from build123d import *

# Parameters (mm, degrees)
F0_W      = 72
F0_H      = 15
F1_DEPTH  = 3.8
F3_DEPTH  = 72
F4_R      = 5
F5_W      = 36
F5_H      = 2
F6_DEPTH  = 1
F7_R      = 0.99999
F10_DEPTH = 4
F11_R     = 2
F12_R     = 1


# Not quite as in the source:
# - a fillet or chamfer is up to 0.001 mm smaller than in the source, because OpenCascade refuses the exact size
# - a pattern or mirror of a feature is missing from the dataset's text; its kind, count and spacing are read off the source's solid


with BuildPart() as f1:
    # F0 (on Top) → F1 (new body)
    with BuildSketch(Plane.XY):
        Rectangle(F0_W, F0_H)
    extrude(amount=F1_DEPTH)

    # F2 (on face) → F3 (join)
    with BuildSketch(Plane.YZ.offset(36)):
        with BuildLine():
            Line((7.5, 7), (5.4598534779, 7))
            ThreePointArc((5.4598534779, 7), (0, 4.8), (-5.4598534779, 7))
            Line((-5.4598534779, 7), (-7.5, 7))
            Line((-7.5, 7), (-7.5, 3.8))
            Line((-7.5, 3.8), (7.5, 3.8))
            Line((7.5, 3.8), (7.5, 7))
        make_face()
    extrude(amount=-F3_DEPTH)

    # F4
    f4_edges = [f1.edges().sort_by_distance(p)[0] for p in [
        (-36, -7.5, 3.5),
        (36, -7.5, 3.5),
        (36, 7.5, 3.5),
        (-36, 7.5, 3.5),
    ]]
    fillet(f4_edges, radius=F4_R)

    # F5 (on face) → F6 (cut)
    with BuildSketch(Plane(origin=(0, 0, 0), x_dir=(1, 0, 0), z_dir=(0, 0, -1))):
        Rectangle(F5_W, F5_H)
    extrude(amount=-F6_DEPTH, mode=Mode.SUBTRACT)

    # F7 (radius 1 in the source; OpenCascade refuses exactly that, so slightly less here)
    f7_edges = [f1.edges().sort_by_distance(p)[0] for p in [
        (0, -1, 1),
        (0, 1, 1),
    ]]
    fillet(f7_edges, radius=F7_R)

    # F9 (on offset) → F10 (cut)
    with BuildSketch(Plane.YZ.offset(16)):
        Polygon((-3.8, 0), (-1.8, 0), (-1.8, 1.8), (0, 1.8), (1.8, 1.8), (1.8, 0), (3.8, 0), (3.8, 3.8), (0, 3.8), (-3.8, 3.8), align=None)
    f10 = extrude(amount=-F10_DEPTH, mode=Mode.SUBTRACT)

    # F10_copies: F10 across plane
    add(f10.mirror(Plane(origin=(0, 0, 0), x_dir=(0, 0, -1), z_dir=(-1, 0, 0))), mode=Mode.SUBTRACT)

    # F11
    f11_edges = [f1.edges().sort_by_distance(p)[0] for p in [
        (14, -3.8, 3.8),
        (14, 3.8, 3.8),
        (-14, -3.8, 3.8),
        (-14, 3.8, 3.8),
    ]]
    fillet(f11_edges, radius=F11_R)

    # F12
    f12_edges = [f1.edges().sort_by_distance(p)[0] for p in [
        (14, -1.8, 1.8),
        (14, 1.8, 1.8),
        (-14, 1.8, 1.8),
        (-14, -1.8, 1.8),
    ]]
    fillet(f12_edges, radius=F12_R)


solid = f1.part
The model under review builds one solid part; all positions refer to its coordinate system, in mm. A direction names the side the tool comes from. Round coordinates to 2 decimals unless told otherwise and drop trailing zeros. Write each loop counter-clockwise with the first axis right and the second up, starting at its lowest first coordinate (ties: lowest second). Pieces come first, ordered by that corner, then holes. Notation, with made-up numbers: M 38.5,63 L 90.5,63 A23 ccw 90.5,99 Z; hole C -16,29.25 d9. An arc over 180 degrees is marked long. Answer as CSV lines item,"result". Start each with the question number.
Q1. Wall thickness on line 1 along X through (y, z) = (-1.75, 2.25); line 2 along Y through (x, z) = (-18, 6.25); line 3 along Y through (x, z) = (17.5, 5.75): over which ranges is each line inside the solid? List them lowest first.
Q2. Tool access review of faces 1 (the face through (14, -3.8, 1)), 2 (the face through (36, 0, 3)), 3 (the face through (-14, 0, 3.8)): name each direction out of +Z, -Z, +X, -X, +Y, -Y from which nothing blocks a thin tool from reaching the whole face with its end or side.
Q3. Consider section D-D, the plane y = -4.5. Give the boundary of the cut face in (x, z).
Q4. Clearance check with flat-ended pins moving along their axes: P1, Ø2, axis at y = 5, z = 4, coming from the -X side; P2, Ø1.3, axis at x = 14, y = 0, coming from the +Z side; P3, Ø1.8, axis at x = -14.5, y = 0, coming from the +Z side. State where each tip first meets the part, or that it passes through.
Q5. The part is to be moulded in two halves that separate along X. For faces 4 (the face through (-34.57, 6, 3.55)), 5 (the face through (14, 3.8, 1)), 6 (the face through (0, -6, 7)), 7 (the face through (16, 0, 2)), say which applies: +X half, -X half, draft (parallel to the pull), parting line (faces both ways), or undercut.
Q6. Consider section B-B, the plane x = -24. Give the boundary of the cut face in (y, z) (3 decimals), then the cut area to 3 significant figures.
Q7. Consider section A-A, the plane z = 3. Give the boundary of the cut face in (x, y).
Result set:
1,line 1,"x = -36 to -16, -12 to 12, 16 to 36"
1,line 2,"y = -7.5 to -4.55, 4.55 to 7.5"
1,line 3,"y = -7.5 to -3.75, 3.75 to 7.5"
2,face 1,"-Z"
2,face 2,"+Z, -Z, +X, +Y, -Y"
2,face 3,"none"
3,outline,"M -35.58,0 L 35.58,0 L 35.58,6.21 L -35.58,6.21 Z"
4,P1,"stops at x = -35.77"
4,P2,"stops at z = 4.83"
4,P3,"stops at z = 4.85"
5,face 4,"-X half"
5,face 5,"undercut"
5,face 6,"draft"
5,face 7,"undercut"
6,outline,"M -7.5,0 L 7.5,0 L 7.5,7 L 5.46,7 A7.875 cw -5.46,7 L -7.5,7 Z"
6,area,"88.5 mm²"
7,outline,"M -36,-2.5 A5 ccw -31,-7.5 L 31,-7.5 A5 ccw 36,-2.5 L 36,2.5 A5 ccw 31,7.5 L -31,7.5 A5 ccw -36,2.5 Z; hole M -16,-3.4 L -12,-3.4 L -12,3.4 L -16,3.4 Z; hole M 12,-3.4 L 16,-3.4 L 16,3.4 L 12,3.4 Z"
